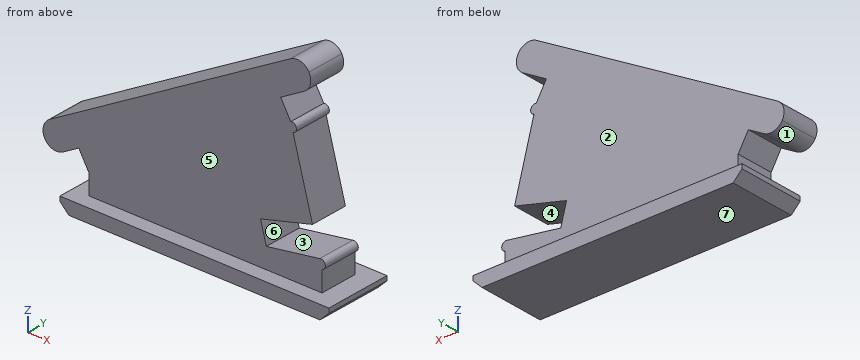
from build123d import *

# Parameters (mm, degrees)
F1_DEPTH = 3.75
F2_DEPTH = 2.125
F3_SIZE  = 1


# Not quite as in the source:
# - a feature names something its author has since deleted; it is built from what else it names


with BuildPart() as f1:
    # F0 (on Front) → F1 (new body, symmetric)
    with BuildSketch(Plane.XZ):
        Polygon((-22.420435602, 1.5), (-24.2496415957, 1.5), (-24.2496415957, 0), (5.7503584043, 0), (5.7503584043, 1.5), (3.579564398, 1.5), align=None)
    extrude(amount=F1_DEPTH, both=True)

    # F0 (on Front) → F2 (join, symmetric)
    with BuildSketch(Plane.XZ):
        with BuildLine():
            Line((-23.545435602, 5.6985571585), (-22.420435602, 3.75))
            Line((-22.420435602, 3.75), (0.0962248963, 16.75))
            Line((0.0962248963, 16.75), (-1.0287751037, 18.6985571585))
            Line((-1.0287751037, 18.6985571585), (1.5693069281, 20.1985605189))
            ThreePointArc((1.5693069281, 20.1985605189), (2.2681808156, 21.1093697133), (2.1183275727, 22.2475885433))
            Line((2.1183275727, 22.2475885433), (2.117101021, 22.2497129931))
            ThreePointArc((2.117101021, 22.2497129931), (1.2027410199, 22.9495484169), (0.0617075083, 22.7950610152))
            Line((0.0617075083, 22.7950610152), (-26.7819009783, 7.2968964295))
            ThreePointArc((-26.7819009783, 7.2968964295), (-27.4812661607, 6.3843043976), (-27.329090085, 5.2446648418))
            Line((-27.329090085, 5.2446648418), (-27.3278673466, 5.242558978))
            ThreePointArc((-27.3278673466, 5.242558978), (-26.4171243137, 4.5463872777), (-25.2806782399, 4.6967143544))
            Line((-25.2806782399, 4.6967143544), (-23.545435602, 5.6985571585))
        make_face()
        Polygon((0.0962248963, 16.75), (-22.420435602, 3.75), (-2.6320926845, 3.75), (-3.2791402973, 6.1648145657), (2.5164146605, 7.7177288363), (0.3550439415, 15.7840741737), align=None)
        Polygon((-22.420435602, 3.75), (-22.420435602, 1.5), (3.579564398, 1.5), (3.579564398, 3.75), (-2.6320926845, 3.75), align=None)
        Polygon((-2.6320926845, 3.75), (3.579564398, 3.75), (3.3207453529, 4.7159258263), align=None)
        with BuildLine():
            Line((3.3207453529, 4.7159258263), (3.579564398, 3.75))
            ThreePointArc((3.579564398, 3.75), (3.9331177885, 4.3623724357), (3.3207453529, 4.7159258263))
        make_face()
        with BuildLine():
            ThreePointArc((0.3550439415, 15.7840741737), (0.708597332, 16.3964466094), (0.0962248963, 16.75))
            Line((0.0962248963, 16.75), (0.3550439415, 15.7840741737))
        make_face()
    extrude(amount=F2_DEPTH, both=True)

    # F3
    f3_edges = [f1.edges().sort_by_distance(p)[0] for p in [
        (-24.249642, 0, 0),
        (5.750358, 0, 0),
    ]]
    chamfer(f3_edges, length=F3_SIZE)


solid = f1.part
The model under review builds one solid part; all positions refer to its coordinate system, in mm. Face numbers are marked on the shaded views. A direction names the side the tool comes from. Round coordinates to 2 decimals unless told otherwise and drop trailing zeros. Loops run counter-clockwise (first coordinate to the right, second up) from the corner with the lowest first, then second, coordinate; pieces in that order, holes last. Notation, with made-up numbers: (-12.75, 43) -> (14.25, 43) arc R19 ccw to (14.25, 61) -> close; hole circle Ø10 at (33, -2). An arc over 180 degrees is marked (long way). Return JSON: item names as keys, results as strings.
(1) Add section C-C on z = 2.5. Write out the cut boundary in (x, y) (3 decimals), plus the area to 4 significant figures.
Solved:
{"outline": "(-22.42, -2.125) -> (3.58, -2.125) -> (3.58, 2.125) -> (-22.42, 2.125) -> close", "area": "110.5 mm2"}
(2) For line 1 (Y direction, x = -10, z = 5) (3 decimals); line 2 (Z direction, x = -13, y = -3.5); line 3 (X direction, y = -1, z = 2), list the stretches that pass through material, from the lowest coordinate up.
Solved:
{"line 1": "-2.125 to 2.125", "line 2": "0 to 1.5", "line 3": "-22.42 to 3.58"}
(3) Add section D-D on y = 3.25. Write out the cut boundary in (x, z).
Solved:
{"outline": "(-24.25, 1) -> (-23.25, 0) -> (4.75, 0) -> (5.75, 1) -> (5.75, 1.5) -> (-24.25, 1.5) -> close"}
(4) The part is to be moulded in two halves that separate along Z. For the marked faces 1, 2 and 3, say which applies: released by +Z, released by -Z, zero draft, split by the parting line, or undercut.
Solved:
{"face 1": "released by -Z", "face 2": "zero draft", "face 3": "undercut"}
(5) Add section B-B on x = -7. Write out the cut boundary in (y, z) (3 decimals), plus the area to 3 significant figures.
Solved:
{"outline": "(-3.75, 0) -> (3.75, 0) -> (3.75, 1.5) -> (2.125, 1.5) -> (2.125, 18.718) -> (-2.125, 18.718) -> (-2.125, 1.5) -> (-3.75, 1.5) -> close", "area": "84.4 mm2"}
(6) For the marked faces 4, 5, 6 and 7, list the 3-axis set-ups (+Z, -Z, +X, -X, +Y, -Y) from which the entire face can be reached by the end or side of a thin tool; tool diameter is ignored.
Solved:
{"face 4": "+X, +Y, -Y", "face 5": "+Z, +X, -X, -Y", "face 6": "+Y, -Y", "face 7": "-Z, +X, -X, +Y, -Y"}
(7) For pin 1 (6.5 mm diameter, centred on x = -10.5, z = 14, fed in from -Y) (3 decimals); pin 2 (0.7 mm diameter, centred on y = 0, z = 3, fed in from +X); pin 3 (2.5 mm diameter, centred on y = -1, z = 2.5, fed in from -X), all flat-tipped, find the tip position at first contact; note any pin that passes through.
Solved:
{"pin 1": "y = -2.125", "pin 2": "x = 3.58", "pin 3": "x = -24.25"}
